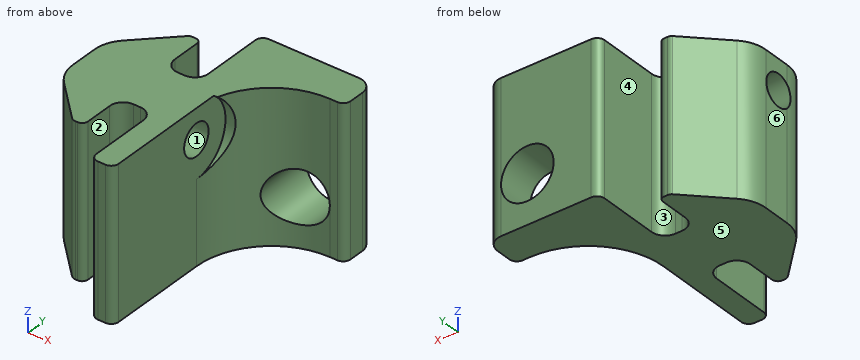
```python
from build123d import *

# Parameters (mm, degrees)
BOSS_EXTRUDE1_DEPTH = 20
SKETCH2_R           = 3.5
CUT_EXTRUDE1_DEPTH  = 65.034014806
SKETCH3_R           = 2.1
CUT_EXTRUDE2_DEPTH  = 43.075221337
SKETCH4_R           = 5
CUT_EXTRUDE3_DEPTH  = 20


with BuildPart() as part:
    # Sketch1 → Boss-Extrude1 (new body)
    with BuildSketch(Plane.XY):
        with BuildLine():
            Line((38.3, 9.881410941), (38.3, 10.745623604))
            Line((38.3, 10.745623604), (38.3, 13.469803951))
            ThreePointArc((38.3, 13.469803951), (37.780173115, 14.724777066), (36.5252, 15.244603951))
            Line((36.5252, 15.244603951), (35.610800366, 15.244603951))
            ThreePointArc((35.610800366, 15.244603951), (34.355826992, 14.724776959), (33.836, 13.469803585))
            Line((33.836, 13.469803585), (33.836, 9.738724213))
            ThreePointArc((33.836, 9.738724213), (33.608795638, 9.190204362), (33.060275787, 8.963))
            Line((33.060275787, 8.963), (32.786933649, 8.963))
            ThreePointArc((32.786933649, 8.963), (32.409953896, 9.037986056), (32.090366071, 9.25152824))
            Line((32.090366071, 9.25152824), (27.33900161, 14.002904388))
            ThreePointArc((27.33900161, 14.002904388), (26.352731832, 15.478964368), (26.0064, 17.220094864))
            Line((26.0064, 17.220094864), (26.0064, 20.879905136))
            ThreePointArc((26.0064, 20.879905136), (26.352731832, 22.621035632), (27.33900161, 24.097095612))
            Line((27.33900161, 24.097095612), (32.177090071, 28.935195973))
            ThreePointArc((32.177090071, 28.935195973), (32.400617966, 29.084552836), (32.664287242, 29.137))
            Line((32.664287242, 29.137), (33.147, 29.137))
            ThreePointArc((33.147, 29.137), (33.634196572, 28.935196572), (33.836, 28.448))
            Line((33.836, 28.448), (33.836, 24.630196049))
            ThreePointArc((33.836, 24.630196049), (34.355826885, 23.375222934), (35.6108, 22.855396049))
            Line((35.6108, 22.855396049), (36.525200183, 22.855396049))
            ThreePointArc((36.525200183, 22.855396049), (37.780173169, 23.37522288), (38.3, 24.630195866))
            Line((38.3, 24.630195866), (38.3, 27.353495632))
            Line((38.3, 27.353495632), (38.3, 28.215588568))
            Line((38.3, 28.215588568), (38.3, 32.710978016))
            ThreePointArc((38.3, 32.710978016), (38.592893219, 33.418084798), (39.3, 33.710978016))
            Line((39.3, 33.710978016), (41.3, 33.710978016))
            Line((41.3, 33.710978016), (51.3, 33.710978016))
            ThreePointArc((51.3, 33.710978016), (52.714213562, 33.125191579), (53.3, 31.710978016))
            Line((53.3, 31.710978016), (53.3, 29.710978016))
            ThreePointArc((53.3, 29.710978016), (53.007106781, 29.003871235), (52.3, 28.710978016))
            Line((52.3, 28.710978016), (51.3, 28.710978016))
            ThreePointArc((51.3, 28.710978016), (44.228932188, 25.782045828), (41.3, 18.710978016))
            Line((41.3, 18.710978016), (41.3, 5.394343623))
            ThreePointArc((41.3, 5.394343623), (41.007106781, 4.687236842), (40.3, 4.394343623))
            Line((40.3, 4.394343623), (39.3, 4.394343623))
            ThreePointArc((39.3, 4.394343623), (38.592893219, 4.687236842), (38.3, 5.394343623))
            Line((38.3, 5.394343623), (38.3, 9.881410941))
        make_face()
    extrude(amount=-BOSS_EXTRUDE1_DEPTH)

    # Sketch2 → Cut-Extrude1 (cut, through all)
    with BuildSketch(Plane(origin=(0, 33.710978016, 0), x_dir=(1, 0, 0), z_dir=(0, 1, 0))):
        with Locations((47.8, 13.5)):
            Circle(SKETCH2_R)
    extrude(amount=-CUT_EXTRUDE1_DEPTH, mode=Mode.SUBTRACT)

    # Sketch3 → Cut-Extrude2 (cut, through all)
    with BuildSketch(Plane(origin=(41.3, 0, 0), x_dir=(0, 0, -1), z_dir=(1, 0, 0))):
        with Locations((4, 18.710978016)):
            Circle(SKETCH3_R)
    extrude(amount=-CUT_EXTRUDE2_DEPTH, mode=Mode.SUBTRACT)

    # Sketch4 → Cut-Extrude3 (cut)
    with BuildSketch(Plane.ZY.offset(-41.3)):
        with Locations((-4, 18.710978016)):
            Circle(SKETCH4_R)
    extrude(amount=-CUT_EXTRUDE3_DEPTH, mode=Mode.SUBTRACT)


solid = part.part
```
Model file for the job. Use its own axes, mm. Face numbers are marked on the shaded views. A direction names the side the tool comes from. Give positions to 0.01 mm unless a question says otherwise; leave off trailing zeros. Loops run counter-clockwise (first coordinate to the right, second up) from the corner with the lowest first, then second, coordinate; pieces in that order, holes last. Notation, with made-up numbers: (49, -16.75) -> (53, -16.75) arc R15 ccw to (53, 0.25) -> close; hole circle Ø10 at (50, -23). An arc over 180 degrees is marked (long way). Use CSV: the item, a comma, the result in double quotes. Start each with the question number.
1) Flat gauge pins, fed straight in: pin 1 Ø6 at (x, z) = (30, -13) entering from +Y; pin 2 Ø1.5 at (y, z) = (26.5, -16.5) entering from +X; pin 3 Ø4 at (y, z) = (11, -11.5) entering from +X. Where does each tip first touch, or does it go through?
2) Slice it at C-C on x = 39.75. Give the cut face in (y, z), plus the area to 3 significant figures.
3) Mould opens along X. For the marked faces 4, 5 and 6 say: released by +X, released by -X, zero draft, split by the parting line, or undercut.
4) Slice it at A-A on x = 45.25. Give the cut face in (y, z).
5) Slice it at B-B on y = 26.5. Give the cut face in (x, z).
6) Wall check: line 1 (X direction, y = 30.25, z = -13.5); line 2 (Z direction, x = 47.8, y = 29.5); line 3 (X direction, y = 17, z = -13). Give the ranges that are in metal, low to high.
7) Tool access for the marked faces 1, 2 and 3: list every direction of +Z, -Z, +X, -X, +Y, -Y with a clear straight run to the whole face (end or side of a thin tool).
Computed values:
1,pin 1,"stops at y = 29.14"
1,pin 2,"stops at x = 46.09"
1,pin 3,"stops at x = 41.3"
2,outline,"(4.39, -20) -> (33.71, -20) -> (33.71, 0) -> (4.39, 0) -> close; hole circle Ø4.2 at (18.71, -4)"
2,area,"572 mm^2"
3,face 4,"undercut"
3,face 5,"zero draft"
3,face 6,"released by -X"
4,outline,"(26.67, -20) -> (33.71, -20) -> (33.71, -15.9) -> (26.67, -15.9) -> close; (26.67, -11.1) -> (33.71, -11.1) -> (33.71, 0) -> (26.67, 0) -> close"
5,outline,"(29.74, -20) -> (33.84, -20) -> (33.84, 0) -> (29.74, 0) -> close; (38.3, -20) -> (45.03, -20) -> (45.03, -15.64) arc R3.5 cw to (45.03, -11.36) -> (45.03, 0) -> (38.3, 0) -> close"
6,line 1,"x = 38.3 to 44.3, 51.3 to 53.3"
6,line 2,"z = -20 to -17, -10 to 0"
6,line 3,"x = 26.01 to 41.3"
7,face 1,"+X, -X"
7,face 2,"+Z, -Z, -Y"
7,face 3,"+Z, -Z, +Y"
